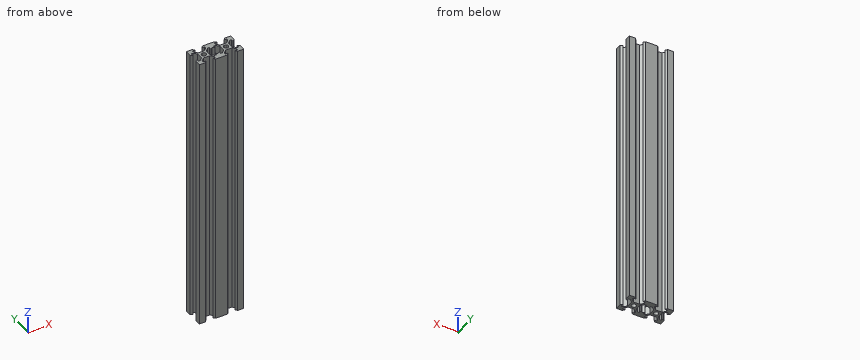
```python
from build123d import *

# Parameters (mm, degrees)
BOSS_EXTRUDE1_DEPTH = 250


with BuildPart() as part:
    # Sketch2 → Boss-Extrude1 (new body)
    with BuildSketch(Plane.XY):
        with BuildLine():
            Line((2.839339828, 3.9), (0, 3.9))
            Line((0, 3.9), (0, 2.1))
            ThreePointArc((0, 2.1), (1.48492424, 1.48492424), (2.1, 0))
            ThreePointArc((2.1, 0), (0, -2.1), (-2.1, 0))
            Line((-2.1, 0), (-3.9, 0))
            Line((-3.9, 0), (-3.9, -2.839339828))
            Line((-3.9, -2.839339828), (-6.560660172, -5.5))
            Line((-6.560660172, -5.5), (-8.2, -5.5))
            Line((-8.2, -5.5), (-8.2, -3.125))
            Line((-8.2, -3.125), (-10, -4.58))
            Line((-10, -4.58), (-10, -10))
            Line((-10, -10), (-4.58, -10))
            Line((-4.58, -10), (-3.125, -8.2))
            Line((-3.125, -8.2), (-5.5, -8.2))
            Line((-5.5, -8.2), (-5.5, -6.560660172))
            Line((-5.5, -6.560660172), (-2.839339828, -3.9))
            Line((-2.839339828, -3.9), (0, -3.9))
            Line((0, -3.9), (2.839339828, -3.9))
            Line((2.839339828, -3.9), (5.5, -6.560660172))
            Line((5.5, -6.560660172), (5.5, -8.2))
            Line((5.5, -8.2), (3.125, -8.2))
            Line((3.125, -8.2), (4.58, -10))
            Line((4.58, -10), (10, -10))
            Line((10, -10), (10, -4.58))
            Line((10, -4.58), (8.2, -3.125))
            Line((8.2, -3.125), (8.2, -5.5))
            Line((8.2, -5.5), (6.560660172, -5.5))
            Line((6.560660172, -5.5), (3.9, -2.839339828))
            Line((3.9, -2.839339828), (3.9, 0))
            Line((3.9, 0), (3.9, 2.839339828))
            Line((3.9, 2.839339828), (6.560660172, 5.5))
            Line((6.560660172, 5.5), (8.2, 5.5))
            Line((8.2, 5.5), (8.2, 3.125))
            Line((8.2, 3.125), (10, 4.58))
            Line((10, 4.58), (10, 10))
            Line((10, 10), (4.58, 10))
            Line((4.58, 10), (3.125, 8.2))
            Line((3.125, 8.2), (5.5, 8.2))
            Line((5.5, 8.2), (5.5, 6.560660172))
            Line((5.5, 6.560660172), (2.839339828, 3.9))
        make_face()
        with BuildLine():
            Line((-1.48492424, 1.48492424), (-10, 10))
            Line((-10, 10), (-10, 4.58))
            Line((-10, 4.58), (-8.2, 3.125))
            Line((-8.2, 3.125), (-8.2, 5.5))
            Line((-8.2, 5.5), (-6.560660172, 5.5))
            Line((-6.560660172, 5.5), (-3.9, 2.839339828))
            Line((-3.9, 2.839339828), (-3.9, 0))
            Line((-3.9, 0), (-2.1, 0))
            ThreePointArc((-2.1, 0), (-1.940147018, 0.803635208), (-1.48492424, 1.48492424))
        make_face()
        with BuildLine():
            Line((-5.5, 6.560660172), (-5.5, 8.2))
            Line((-5.5, 8.2), (-3.125, 8.2))
            Line((-3.125, 8.2), (-4.58, 10))
            Line((-4.58, 10), (-10, 10))
            Line((-10, 10), (-1.48492424, 1.48492424))
            ThreePointArc((-1.48492424, 1.48492424), (-0.803635208, 1.940147018), (0, 2.1))
            Line((0, 2.1), (0, 3.9))
            Line((0, 3.9), (-2.839339828, 3.9))
            Line((-2.839339828, 3.9), (-5.5, 6.560660172))
        make_face()
    boss_extrude1 = extrude(amount=BOSS_EXTRUDE1_DEPTH)

    # Mirror1: Boss-Extrude1 across plane
    add(boss_extrude1.mirror(Plane(origin=(10, 0, 250), x_dir=(0, 0, 1), z_dir=(1, 0, 0))))


solid = part.part
```
Read the model definition and answer for the solid it produces. Units are mm, in the model's axes. Coordinates: 2 decimals unless noted, no trailing zeros. Answer as a JSON object with one key per item and string values. Group by question number.
1. Consider L1, parallel to X at y = 8.25, z = 146; L2, parallel to X at y = 3.5, z = 10.5; L3, parallel to Y at x = 10, z = 11.5. Determine where each line is inside the solid, lowest interval first. Write a range as [from, to].
2. Each of these flat-tipped pins is pushed along its axis until it touches: P1, Ø1.9, axis at y = -4, z = 108.5, coming from the +X side; P2, Ø3, axis at x = 1, z = 165.5, coming from the -Y side; P3, Ø3, axis at y = 0, z = 184.5, coming from the +X side. Where does it stop, or does it pass through?
3. A cutting plane is placed at A-A (z = 30.5). Give the number of separate pieces and of enclosed holes in the cut face, plus the area to 3 significant figures.
Worked out:
{
 "1": {"L1": "x = [-10, -3.17], [3.17, 16.83], [23.17, 30]", "L2": "x = [-8.66, -8.2], [-4.56, 4.56], [8.2, 8.66], [11.34, 11.8], [15.44, 24.56], [28.2, 28.66]", "L3": "y = [-10, -4.58], [4.58, 10]"},
 "2": {"P1": "stops at x = 30", "P2": "stops at y = -3.9", "P3": "stops at x = 23.9"},
 "3": {"separate pieces": "1", "enclosed holes": "3", "area": "340 mm²"}
}
